Input: part model. Units: mm. Frame: model coordinates. Face numbers are marked on the shaded views. A direction names the side the tool comes from. Round coordinates to 2 decimals unless told otherwise and drop trailing zeros. Order: outer loops, then holes, each group sorted by start corner. A loop starts at its lowest first (then second) coordinate and runs counter-clockwise, first axis right, second up. Notation, with made-up numbers: (7.25, 26.5) -> (63.25, 26.5) arc R5 cw to (63.25, 35.5) -> close; hole circle Ø10 at (24.5, -35.5). An arc over 180 degrees is marked (long way). Answer as CSV lines item,"result". Start each with the question number.
1) First-contact query: P1, Ø6, axis at x = 1.5, y = 14.5, coming from the +Z side. Flat tip, straight axial feed; report the tip coordinate or a pass-through.
2) Section query C-C, the plane z = 2.55. Output: boundary loops of the cut face in (x, y), and give its area (3 significant figures).
3) Section query A-A, the plane z = 4.1. Output: boundary loops of the cut face in (x, y), and give its area (3 significant figures).
4) Mould query, pull axis X, two halves, no side actions, for the marked faces 3, 4, 5 and 6. Classes: +X half, -X half, draft (parallel to the pull), parting line (faces both ways), or undercut.
5) Line query: L1, parallel to Y at x = 0, z = 1.9; L2, parallel to Y at x = 12, z = 3.3; L3, parallel to Y at x = 12, z = 2.8. Output: solid intervals per line, ascending.
6) Section query B-B, the plane z = 0.65. Output: boundary loops of the cut face in (x, y), and give its area (3 significant figures).
7) Section query D-D, the plane y = 15.75. Output: boundary loops of the cut face in (x, z), and give its area (3 significant figures).
8) Access query for the marked faces 1 and 2. Directions: +Z, -Z, +X, -X, +Y, -Y. A direction counts if a zero-diameter tool reaches every point of the face in a straight line with its end or side. Return the directions, or none.
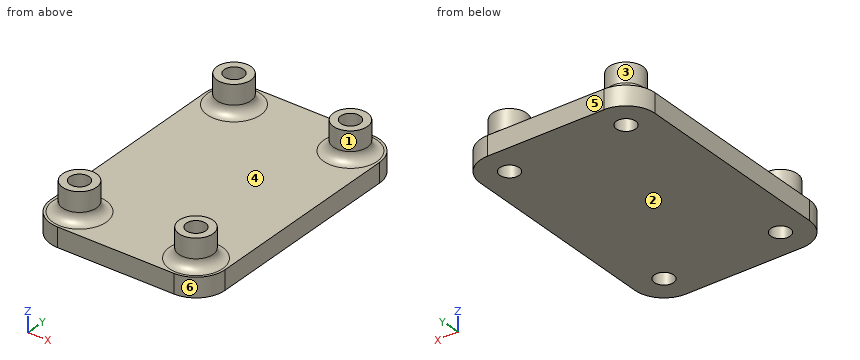
Autodesk Inventor part; units mm, degrees
ref_plane "YZ Plane" through (0, 0, 0) normal (1, 0, 0) x (0, 1, 0)
ref_plane "XZ Plane" through (0, 0, 0) normal (0, 1, 0) x (-1, 0, 0)
ref_plane "XY Plane" through (0, 0, 0) normal (0, 0, 1) x (1, 0, 0)
sketch "Náčrt1" plane through (0, 0, 0) normal (0, 0, 1) x (1, 0, 0)
  circle A0 centre (0, 0) radius 1
  circle A1 centre (12, 0) radius 1
  circle A2 centre (0, 21) radius 1
  circle A3 centre (12, 21) radius 1
  line L0 (12, 24) -> (0, 24)
  arc A4 (0, 24) -> (-3, 21) centre (0, 21) ccw
  line L1 (-3, 21) -> (-3, 0)
  arc A5 (-3, 0) -> (0, -3) centre (0, 0) ccw
  line L2 (0, -3) -> (12, -3)
  arc A6 (12, -3) -> (15, 0) centre (12, 0) ccw
  line L3 (15, 0) -> (15, 21)
  arc A7 (15, 21) -> (12, 24) centre (12, 21) ccw
  dimension "d0" = 2
  dimension "d1" = 10
extrude "Vysunutí1" add sketch "Náčrt1" along normal blind 2
sketch "Náčrt2" plane through (0, 0, 2) normal (0, 0, 1) x (1, 0, 0)
  circle A0 centre (0, 0) radius 1
  circle A1 centre (0, 0) radius 1
  line L0 (0, -3) -> (12, -3)
  circle A2 centre (12, 0) radius 1
  line L1 (-3, 21) -> (-3, 0)
  line L2 (15, 0) -> (15, 21)
  circle A3 centre (0, 21) radius 1
  circle A4 centre (12, 21) radius 1
  circle A5 centre (0, 21) radius 1.75
  circle A6 centre (12, 21) radius 1.75
  circle A7 centre (12, 0) radius 1.75
  circle A8 centre (0, 0) radius 1.75
  dimension "d10" = 0.75
  dimension "d11" = 0.75
  dimension "d12" = 0.75
  dimension "d14" = 0.75
extrude "Vysunutí2" add sketch "Náčrt2" along normal blind 3
fillet "Zaoblení1" radius 1 1 edges at (-1.75, 0, 2)
fillet "Zaoblení2" radius 1 3 edges at (-1.75, 21, 2) (10.25, 21, 2) (10.25, 0, 2)
properties part number "drzak_kamery"
Findings:
1,P1,"stops at z = 2"
2,outline,"circle Ø3.71 at (0, 0); circle Ø3.71 at (0, 21); circle Ø3.71 at (12, 0); circle Ø3.71 at (12, 21); hole circle Ø2 at (0, 0); hole circle Ø2 at (0, 21); hole circle Ø2 at (12, 0); hole circle Ø2 at (12, 21)"
2,area,"30.8 mm^2"
3,outline,"circle Ø3.5 at (0, 0); circle Ø3.5 at (0, 21); circle Ø3.5 at (12, 0); circle Ø3.5 at (12, 21); hole circle Ø2 at (0, 0); hole circle Ø2 at (0, 21); hole circle Ø2 at (12, 0); hole circle Ø2 at (12, 21)"
3,area,"25.9 mm^2"
4,face 3,"undercut"
4,face 4,"undercut"
4,face 5,"draft"
4,face 6,"+X half"
5,L1,"y = -3 to -1, 1 to 20, 22 to 24"
5,L2,"y = -1.75 to -1, 1 to 1.75, 19.25 to 20, 22 to 22.75"
5,L3,"y = -1.77 to -1, 1 to 1.77, 19.23 to 20, 22 to 22.77"
6,outline,"(-3, 0) arc R3 ccw to (0, -3) -> (12, -3) arc R3 ccw to (15, 0) -> (15, 21) arc R3 ccw to (12, 24) -> (0, 24) arc R3 ccw to (-3, 21) -> close; hole circle Ø2 at (0, 0); hole circle Ø2 at (0, 21); hole circle Ø2 at (12, 0); hole circle Ø2 at (12, 21)"
6,area,"466 mm^2"
7,outline,"(-3, 0) -> (15, 0) -> (15, 2) -> (-3, 2) -> close"
7,area,"36.0 mm^2"
8,face 1,"+Z"
8,face 2,"-Z, +X, -X, +Y, -Y"
